from build123d import *

# Parameters (mm, degrees)
SKETCH1_W           = 55
SKETCH1_H           = 55
SKETCH1_R           = 4.1
BOSS_EXTRUDE1_DEPTH = 9.525
SKETCH1_3_R         = 4.1
SKETCH1_3_R_2       = 2.2
BOSS_EXTRUDE2_DEPTH = 4.525
SKETCH3_R           = 3.0127
CUT_EXTRUDE1_DEPTH  = 79.362782142
SKETCH5_R           = 3.2512
CUT_EXTRUDE2_DEPTH  = 6.4008
CHAMFER1_SIZE       = 0.5
SKETCH6_R           = 1.25
CUT_EXTRUDE3_DEPTH  = 79.362782142
CHAMFER2_SIZE       = 0.5


with BuildPart() as part:
    # Sketch1 → Boss-Extrude1 (new body)
    with BuildSketch(Plane.XY):
        with Locations((27.5, 27.5)):
            Rectangle(SKETCH1_W, SKETCH1_H)
        with Locations(Location((37.5, 27.5, 0), (0, 0, 180))):
            Circle(SKETCH1_R, mode=Mode.SUBTRACT)
        with Locations(Location((17.5, 27.5, 0), (0, 0, 180))):
            Circle(SKETCH1_R, mode=Mode.SUBTRACT)
    extrude(amount=BOSS_EXTRUDE1_DEPTH)

    # Sketch1_3 → Boss-Extrude2 (add)
    # profile 1 of 2: a face of its own
    with BuildSketch(Plane.XY):
        with Locations(Location((17.5, 27.5, 0), (0, 0, 180))):
            Circle(SKETCH1_3_R)
        with Locations(Location((17.5, 27.5, 0), (0, 0, 180))):
            Circle(SKETCH1_3_R_2, mode=Mode.SUBTRACT)
    # profile 2 of 2: a face of its own
    with BuildSketch(Plane.XY):
        with Locations(Location((37.5, 27.5, 0), (0, 0, 180))):
            Circle(SKETCH1_3_R)
        with Locations(Location((37.5, 27.5, 0), (0, 0, 180))):
            Circle(SKETCH1_3_R_2, mode=Mode.SUBTRACT)
    extrude(amount=BOSS_EXTRUDE2_DEPTH)

    # Sketch3 → Cut-Extrude1 (cut, through all)
    with BuildSketch(Plane.XY.offset(9.525)):
        with Locations((27.5, 49)):
            Circle(SKETCH3_R)
        with Locations((6, 27.5)):
            Circle(SKETCH3_R)
        with Locations((49, 27.5)):
            Circle(SKETCH3_R)
        with Locations((27.5, 6)):
            Circle(SKETCH3_R)
    extrude(amount=-CUT_EXTRUDE1_DEPTH, mode=Mode.SUBTRACT)

    # Sketch5 → Cut-Extrude2 (cut)
    with BuildSketch(Plane.XY.offset(9.525)):
        with Locations((6, 49)):
            Circle(SKETCH5_R)
        with Locations((49, 49)):
            Circle(SKETCH5_R)
        with Locations((49, 6)):
            Circle(SKETCH5_R)
        with Locations((6, 6)):
            Circle(SKETCH5_R)
    extrude(amount=-CUT_EXTRUDE2_DEPTH, mode=Mode.SUBTRACT)

    # Chamfer1
    chamfer1_edges = [part.edges().sort_by_distance(p)[0] for p in [
        (21.6, 27.5, 9.525),
        (0, 0, 4.7625),
        (0, 55, 4.7625),
        (55, 55, 4.7625),
        (55, 0, 4.7625),
        (27.5, 0, 9.525),
        (55, 27.5, 9.525),
        (19.7, 27.5, 0),
        (27.5, 55, 9.525),
        (39.7, 27.5, 0),
        (0, 27.5, 9.525),
        (24.4873, 49, 0),
        (24.4873, 49, 9.525),
        (2.9873, 27.5, 0),
        (2.9873, 27.5, 9.525),
        (45.9873, 27.5, 0),
        (45.9873, 27.5, 9.525),
        (24.4873, 6, 0),
        (24.4873, 6, 9.525),
        (2.7488, 49, 9.525),
        (45.7488, 49, 9.525),
        (45.7488, 6, 9.525),
        (2.7488, 6, 9.525),
        (41.6, 27.5, 9.525),
        (0, 27.5, 0),
        (27.5, 55, 0),
        (55, 27.5, 0),
        (27.5, 0, 0),
    ]]
    chamfer(chamfer1_edges, length=CHAMFER1_SIZE)

    # Sketch6 → Cut-Extrude3 (cut, through all)
    with BuildSketch(Plane.XY.offset(9.525)):
        with Locations((6, 49)):
            Circle(SKETCH6_R)
        with Locations((49, 49)):
            Circle(SKETCH6_R)
        with Locations((49, 6)):
            Circle(SKETCH6_R)
        with Locations((6, 6)):
            Circle(SKETCH6_R)
    extrude(amount=-CUT_EXTRUDE3_DEPTH, mode=Mode.SUBTRACT)

    # Chamfer2
    chamfer2_edges = [part.edges().sort_by_distance(p)[0] for p in [
        (4.75, 49, 3.1242),
        (4.75, 49, 0),
        (47.75, 49, 3.1242),
        (47.75, 49, 0),
        (47.75, 6, 3.1242),
        (47.75, 6, 0),
        (4.75, 6, 3.1242),
        (4.75, 6, 0),
    ]]
    chamfer(chamfer2_edges, length=CHAMFER2_SIZE)


solid = part.part
Design review of the part built by this model. Coordinates are the model's own, in mm. A direction names the side the tool comes from. Round coordinates to 2 decimals unless told otherwise and drop trailing zeros. Write each loop counter-clockwise with the first axis right and the second up, starting at its lowest first coordinate (ties: lowest second). Pieces come first, ordered by that corner, then holes. Notation, with made-up numbers: M -13,43 L 8,43 A23 cw 8,73 Z; hole C -31,11 d6. An arc over 180 degrees is marked long. One line per item, written item: value. Start each with the question number.
1. Take a section at C-C on x = 37.5. State the section outline as (y, z) points (3 decimals).
2. Take a section at B-B on x = 27.5. State the section outline as (y, z) points (3 decimals), then the cut area to 3 significant figures.
3. To check wall thickness, follow probe 1 along Y at (x, z) = (6, 1.7); probe 2 along Y at (x, z) = (49, 5.7); probe 3 along X at (y, z) = (47.5, 4). State the ranges of each line that lie inside material, in increasing order. Write a range as from..to.
4. For faces 1 (the face through (48.84, 50.24, 1.58)), 2 (the face through (35.7, 29.3, 4.525)), list the 3-axis set-ups (+Z, -Z, +X, -X, +Y, -Y) from which the entire face can be reached by the end or side of a thin tool; tool diameter is ignored.
5. Clearance check with flat-ended pins moving along their axes: P1, Ø10.5, axis at x = 37.5, y = 27.5, coming from the +Z side (3 decimals); P2, Ø3, axis at x = 6, y = 6, coming from the +Z side; P3, Ø3.5, axis at x = 50, y = 48.5, coming from the +Z side; P4, Ø3.5, axis at x = 50.5, y = 7, coming from the +Z side. State where each tip first meets the part, or that it passes through.
6. Take a section at A-A on z = 6.5. State how many separate pieces and enclosed holes the cut face has, then the cut area to 3 significant figures.
Computed:
1. outline: M 0,0.5 L 0.5,0 L 24.8,0 L 25.3,0.5 L 25.3,4.525 L 23.4,4.525 L 23.4,9.025 L 22.9,9.525 L 0.5,9.525 L 0,9.025 Z; M 29.7,0.5 L 30.2,0 L 54.5,0 L 55,0.5 L 55,9.025 L 54.5,9.525 L 32.1,9.525 L 31.6,9.025 L 31.6,4.525 L 29.7,4.525 Z
2. outline: M 0,0.5 L 0.5,0 L 2.487,0 L 2.987,0.5 L 2.987,9.025 L 2.487,9.525 L 0.5,9.525 L 0,9.025 Z; M 9.013,0.5 L 9.513,0 L 45.487,0 L 45.987,0.5 L 45.987,9.025 L 45.487,9.525 L 9.513,9.525 L 9.013,9.025 Z; M 52.013,0.5 L 52.513,0 L 54.5,0 L 55,0.5 L 55,9.025 L 54.5,9.525 L 52.513,9.525 L 52.013,9.025 Z
2. area: 408 mm²
3. probe 1: y = 0..4.75, 7.25..24.49, 30.51..47.75, 50.25..55
3. probe 2: y = 0..2.75, 9.25..24.49, 30.51..45.75, 52.25..55
3. probe 3: x = 0..3.12, 8.88..24.89, 30.11..46.12, 51.88..55
4. face 1: +Z, -Z
4. face 2: +Z
5. P1: stops at z = 9.525
5. P2: stops at z = 2.87
5. P3: stops at z = 3.12
5. P4: stops at z = 9.33
6. separate pieces: 1
6. enclosed holes: 10
6. area: 2,670 mm²
